Check sheet for the modelled part. Datum: model origin and axes. Units: mm. A direction names the side the tool comes from. Round coordinates to 2 decimals unless told otherwise and drop trailing zeros. Order: outer loops, then holes, each group sorted by start corner. A loop starts at its lowest first (then second) coordinate and runs counter-clockwise, first axis right, second up.
Q1. Cross-section at B-B on y = -29. Record the cut outline in (x, z).
Q2. Scan lines: probe 1 along Y at (x, z) = (-133, 6.25); probe 2 along X at (y, z) = (-55, 3); probe 3 along Y at (x, z) = (-90.5, 1). Record each from-to range of solid material in increasing order.
Q3. Mould release check, pull along X, two halves, no side actions. Record for faces 1 (the flat face through (-46.83, 130.82, 3.13)), 2 (the flat face through (42.943, 47.813, 3.131)), 3 (the flat face through (-137.6, 142, 3.2)), 4 (the flat face through (-214.89, 97.76, 3.13)): +X half, -X half, draft (parallel to the pull), parting line (faces both ways), or undercut.
Q4. Cross-section at A-A on z = 2. Give the number of separate pieces and of enclosed holes in the cut face, then the cut area to 3 significant figures.
Q5. Cross-section at C-C on x = 1.5. Record the cut outline in (y, z).
Q6. Depth check by flat-ended pin: P1, Ø3, axis at x = -78.5, z = 3, coming from the +Y side; P2, Ø3, axis at y = 18, z = 2.5, coming from the +X side; P3, Ø2, axis at x = -165, z = 1, coming from the +Y side. Enter the tip coordinate at first touch or a pass-through.
Q7. Set-up check for faces 5 (the flat face through (-54.39, -31.79, 3.13)), 6 (the cylindrical face through (-63.76, 80.51, 3.13)): record each of +Z, -Z, +X, -X, +Y, -Y from which the full face is reachable in a straight line by a thin tool's end or side.
Autodesk Inventor part; units mm, degrees
ref_plane "YZ Plane" through (0, 0, 0) normal (1, 0, 0) x (0, 1, 0)
ref_plane "XZ Plane" through (0, 0, 0) normal (0, 1, 0) x (-1, 0, 0)
ref_plane "XY Plane" through (0, 0, 0) normal (0, 0, 1) x (1, 0, 0)
sketch "Sketch1" plane through (0, 0, 0) normal (0, 0, 1) x (1, 0, 0)
  circle A0 centre (78.7027, 64.253) radius 50.8 construction
  circle A1 centre (-78.7027, -64.253) radius 50.8 construction
  circle A2 centre (0, 0) radius 50.8 construction
  line L0 (-39.3513, -32.1265) -> (39.3513, 32.1265) construction
  line L1 (78.7027, 64.253) -> (-78.7027, -64.253) construction
  line L2 (-3.7208, 6.6498) -> (-3.7208, 50.6636) construction
  line L3 (-233.7404, -115.053) -> (631.6516, -115.053) construction
  circle A3 centre (140.9799, -57.903) radius 57.15 construction
  circle A4 centre (78.7027, 64.253) radius 14.2621
  circle A5 centre (-78.7027, -64.253) radius 14.2621
  circle A6 centre (-3.7208, 6.6498) radius 57.15 construction
  circle A7 centre (-78.7027, -64.253) radius 30.1371 construction
  circle A8 centre (78.7027, 64.253) radius 30.1371 construction
  circle A9 centre (-45.9582, 108.8109) radius 14.2621
  line L4 (-45.9582, 108.8109) -> (78.7027, 64.253) construction
  circle A10 centre (78.7027, 64.253) radius 14.3256 construction
  circle A11 centre (-78.7027, -64.253) radius 14.3256 construction
  circle A12 centre (-70.3374, 67.8545) radius 14.2621
  line L5 (-78.7027, -64.253) -> (-70.3374, 67.8545) construction
  circle A13 centre (-70.3374, 67.8545) radius 23.8316 construction
  circle A14 centre (-45.9582, 108.8109) radius 23.8316 construction
  line L6 (20.6869, 58.3256) -> (65.8317, 37.0027)
  line L7 (-49.1354, -58.4201) -> (-59.7901, -4.4114)
  arc A15 (20.6869, 58.3256) -> (-59.7901, -4.4114) centre (-3.7208, 6.6498) ccw
  line L8 (-201.842, 171.7522) -> (-176.8279, 167.3416)
  line L9 (-176.8279, 167.3416) -> (-203.2918, 17.2569) construction
  line L10 (-203.2918, 17.2569) -> (-228.306, 21.6675) construction
  line L11 (-228.306, 21.6675) -> (-201.842, 171.7522) construction
  line L12 (-247.3095, -86.1068) -> (28.2095, -134.6882) construction
  line L13 (-202.9446, 165.4987) -> (212.0535, 92.3234) construction
  line L14 (-202.9446, 165.4987) -> (-247.3095, -86.1068) construction
  circle A16 centre (-145.4024, 107.8708) radius 31.75
  line L15 (-71.8434, 44.0706) -> (-75.4924, -13.5546) construction
  circle A17 centre (21.8973, 84.5571) radius 9.525 construction
  line L16 (-189.3349, 169.5469) -> (-215.7989, 19.4622) construction
  line L17 (-192.0916, 153.9131) -> (-213.0422, 35.096) construction
  circle A18 centre (-145.4024, 107.8708) radius 17.4625 construction
  circle A19 centre (-145.4024, 107.8708) radius 9.525
  circle A20 centre (-45.9582, 108.8109) radius 30.1816 construction
  line L18 (-201.842, 171.7522) -> (-228.306, 21.6675)
  arc A21 (65.8317, 37.0027) -> (86.8534, 93.267) centre (78.7027, 64.253) ccw
  arc A22 (-108.4816, -68.8852) -> (-49.1354, -58.4201) centre (-78.7027, -64.253) ccw
  line L19 (-145.4024, 107.8708) -> (-128.993, 113.8433) construction
  line L20 (-111.0919, 120.3588) -> (-179.7129, 95.3828) construction
  circle A23 centre (-179.7129, 95.3828) radius 4.7625 construction
  line L21 (0, 0) -> (-3.7208, 6.6498) construction
  circle A24 centre (78.7027, 64.253) radius 28.6512 construction
  line L22 (66.184, 38.4815) -> (-52.1898, 95.9822) construction
  line L23 (85.3565, 92.1209) -> (-42.6461, 122.6831) construction
  line L24 (-176.8279, 167.3416) -> (86.8534, 93.267)
  line L25 (-145.4024, 107.8708) -> (-121.2984, 36.7761) construction
  circle A25 centre (-121.2984, 36.7761) radius 31.75 construction
  circle A26 centre (-121.2984, 36.7761) radius 14.2621
  line L26 (-70.3374, 67.8545) -> (-121.2984, 36.7761) construction
  circle A27 centre (-145.4024, 107.8708) radius 25.4 construction
  arc A28 (-108.4816, -68.8852) -> (-228.306, 21.6675) centre (-215.1488, -85.4777) ccw
  circle A29 centre (-145.4024, 107.8708) radius 36.5125 construction
  line L27 (-178.494, 123.3016) -> (-145.4024, 107.8708) construction
  point P0 (-73.6679, 15.258)
  point P1 (-202.5669, 94.5046)
  point P2 (-202.5669, 94.5046)
  point P3 (-142.3701, 125.068)
  point P4 (-158.7795, 119.0955)
  point P5 (-161.8118, 101.8983)
  point P6 (-148.4348, 90.6736)
  point P7 (-132.0254, 96.6461)
  point P8 (-121.5342, 116.5581)
  point P9 (-140.9918, 132.8849)
  point P10 (-164.86, 124.1976)
  point P11 (-169.2706, 99.1835)
  point P12 (-149.8131, 82.8567)
  point P13 (-125.9449, 91.544)
  point P14 (-157.8904, 142.1813)
  point P15 (-179.7129, 95.3828)
  point P16 (-132.9144, 73.5603)
  point P17 (-129.9716, 140.9624)
  point P18 (-160.8333, 74.7792)
  point P19 (-112.3109, 92.4399)
  dimension "d7" = 101.6
  dimension "d18" = 47.6631
  dimension "d34" = 34.925
  dimension "d65" = 50.8
  dimension "d3" = 50.772
  dimension "d4" = 0
  dimension "d8" = 101.6
  dimension "d9" = 28.5242
  dimension "d10" = 101.6
  dimension "d11" = 114.3
  dimension "d12" = 114.3
  dimension "d13" = 15.875
  dimension "d14" = 15.875
  dimension "d15" = 132.3848
  dimension "d16" = 28.6512
  dimension "d17" = 132.3721
  dimension "d19" = 47.6631
  dimension "d22" = 25.4
  dimension "d23" = 152.4
  dimension "d26" = 255.4869
  dimension "d27" = 63.5
  dimension "d30" = 203.2
  dimension "d31" = 10
  dimension "d32" = 19.05
  dimension "d33" = 120.65
  dimension "d35" = 19.05
  dimension "d36" = 6.35
  dimension "d40" = 360
  dimension "d44" = 9.525
  dimension "d55" = 80
  dimension "d56" = 7.62
  dimension "d58" = 57.3024
  dimension "d59" = 63.5
  dimension "d60" = 75.0697
  dimension "d61" = 59.69
  dimension "d62" = 55
  dimension "d68" = 360
  dimension "d70" = 41.275
  dimension "d71" = 60
  dimension "d88" = 360
  dimension "d93" = 360
  dimension "d95" = 45
  dimension "d96" = 6.35
  dimension "d97" = 20.955
  dimension "d98" = 107.95
extrude "Extrusion1" add sketch "Sketch1" along normal blind 6.35 contours A15 L7 A22 A28 L18 L8 L24 A21 L6
hole "Hole1" at (21.8973, 84.5571, 0) at (-192.0916, 153.9131, 0) at (-202.5669, 94.5046, 0) at (-213.0422, 35.096, 0) at (-128.993, 113.8433, 0) at (-142.3701, 125.068, 0) at (-158.7795, 119.0955, 0) at (-161.8118, 101.8983, 0) at (-148.4348, 90.6736, 0) at (-132.0254, 96.6461, 0) at (-149.8131, 82.8567, 0) at (-169.2706, 99.1835, 0) at (-164.86, 124.1976, 0) at (-140.9918, 132.8849, 0) at (-121.5342, 116.5581, 0) at (-125.9449, 91.544, 0) at (-73.6679, 15.258, 0) at (-129.9716, 140.9624, 0) at (-178.494, 123.3016, 0) at (-160.8333, 74.7792, 0) at (-112.3109, 92.4399, 0) at (-179.7129, 95.3828, 0) at (-111.0919, 120.3588, 0) direction (0, 0, 1) diameter 5.1054 end through all
sketch "Sketch2" plane through (0, 0, 6.35) normal (0, 0, 1) x (1, 0, 0)
  circle A0 centre (-213.0422, 35.096) radius 2.5527 construction
  circle A1 centre (-192.0916, 153.9131) radius 2.5527 construction
  circle A2 centre (21.8973, 84.5571) radius 2.5527 construction
  circle A3 centre (-202.5669, 94.5046) radius 2.5527 construction
  circle A4 centre (-73.6679, 15.258) radius 2.5527 construction
  line L0 (-49.1354, -58.4201) -> (-59.7901, -4.4114) construction
  arc A5 (20.6869, 58.3256) -> (-59.7901, -4.4114) centre (-3.7208, 6.6498) ccw construction
  line L1 (20.6869, 58.3256) -> (65.8317, 37.0027) construction
  arc A6 (65.8317, 37.0027) -> (86.8534, 93.267) centre (78.7027, 64.253) ccw construction
  line L2 (86.8534, 93.267) -> (-176.8279, 167.3416) construction
  line L3 (-176.8279, 167.3416) -> (-201.842, 171.7522) construction
  line L4 (-201.842, 171.7522) -> (-228.306, 21.6675) construction
  arc A7 (-108.4816, -68.8852) -> (-228.306, 21.6675) centre (-215.1488, -85.4777) ccw construction
  arc A8 (-108.4816, -68.8852) -> (-49.1354, -58.4201) centre (-78.7027, -64.253) ccw construction
  circle A9 centre (-70.3374, 67.8545) radius 14.2621 construction
  circle A10 centre (-121.2984, 36.7761) radius 14.2621 construction
  circle A11 centre (-45.9582, 108.8109) radius 14.2621 construction
  circle A12 centre (-78.7027, -64.253) radius 14.2621 construction
  circle A13 centre (78.7027, 64.253) radius 14.2621 construction
  line L5 (-77.3744, -43.2765) -> (-80.0309, -85.2295) construction
  line L6 (-139.2432, 25.8325) -> (-103.3536, 47.7196) construction
  line L7 (-69.0091, 88.831) -> (-71.6657, 46.878) construction
  line L8 (-65.7504, 115.8853) -> (-26.166, 101.7365) construction
  line L9 (58.9105, 71.3274) -> (98.4948, 57.1787) construction
  circle A14 centre (-70.3374, 67.8545) radius 14.2621 construction
  line L10 (-45.9582, 108.8109) -> (-70.3374, 67.8545) construction
  line L11 (-45.9582, 108.8109) -> (78.7027, 64.253) construction
  line L12 (-70.3374, 67.8545) -> (-121.2984, 36.7761) construction
  line L13 (-70.3374, 67.8545) -> (-78.7027, -64.253) construction
  circle A15 centre (-112.3109, 92.4399) radius 2.5527
  point P0 (0, 0)
  point P1 (-116.0598, 70.5176)
  point P2 (-113.1961, 73.3575)
  dimension "d72" = 42.037
hole "Hole2" at (-77.3744, -43.2765, 6.35) at (-103.3536, 47.7196, 6.35) at (-80.0309, -85.2295, 6.35) at (-139.2432, 25.8325, 6.35) at (-71.6657, 46.878, 6.35) at (-69.0091, 88.831, 6.35) at (-26.166, 101.7365, 6.35) at (-65.7504, 115.8853, 6.35) at (98.4948, 57.1787, 6.35) at (58.9105, 71.3274, 6.35) direction (0, 0, -1) diameter 5.1054 end through all
sketch "Sketch3" plane through (0, 0, 6.35) normal (0, 0, 1) x (1, 0, 0)
  circle A0 centre (-145.4024, 107.8708) radius 31.75
  line L0 (-176.4346, 114.5838) -> (-169.5558, 146.3824)
  line L1 (-169.5558, 146.3824) -> (-151.6546, 152.8979)
  line L2 (-151.6546, 152.8979) -> (-125.9454, 132.9604)
  circle A1 centre (-111.0919, 120.3588) radius 2.5527
  circle A2 centre (-183.1052, 76.1445) radius 2.5527
  line L3 (-105.3056, 104.4612) -> (-183.1052, 76.1445) construction
  line L4 (-183.1052, 76.1445) -> (-139.6162, 91.9732)
  line L5 (-145.4024, 107.8708) -> (-160.6052, 149.6401) construction
  point P0 (0, 0)
  dimension "d80" = 44.45
  dimension "d82" = 19.05
extrude "Extrusion2" cut sketch "Sketch3" against normal through all contours A0 L0 L1 L2
fillet "Fillet1" radius 6.35 2 edges at (-169.5558, 146.3824, 3.175) (-151.6546, 152.8979, 3.175)
properties part number "GP9-002" material "Polycarbonate, Smoke"
Results found:
1. outline: (-123.15, 0) - (-54.94, 0) - (-54.94, 6.35) - (-123.15, 6.35) - close
2. probe 1: y = -15.44 to 28.62, 44.93 to 78.64, 138.43 to 155.03
2. probe 2: x = -111.59 to -89.56, -67.85 to -49.81
2. probe 3: y = -91.98 to -72.27, -56.24 to 143.09
3. face 1: +X half
3. face 2: undercut
3. face 3: undercut
3. face 4: -X half
4. separate pieces: 1
4. enclosed holes: 27
4. area: 32,100 mm2
5. outline: (63.56, 0) - (117.24, 0) - (117.24, 6.35) - (63.56, 6.35) - close
6. P1: stops at y = 140.14
6. P2: stops at x = -59.41
6. P3: stops at y = 164.3
7. face 5: +Z, -Z, +X
7. face 6: +Z, -Z
